Source: three-view drawing plus pictorial views. Frame: mm from the lowest corner of the part. A direction names the side the tool comes from. Give positions to 0.01 mm unless a question says otherwise; leave off trailing zeros. Order: outer loops, then holes, each group sorted by start corner. A loop starts at its lowest first (then second) coordinate and runs counter-clockwise, first axis right, second up.
1) Section D-D, the plane x = 21. Return loops of the section in (y, z), plus the area to 3 significant figures.
2) Access query for the marked faces 1 and 2. Directions: +Z, -Z, +X, -X, +Y, -Y. A direction counts if a zero-diameter tool reaches every point of the face in a straight line with its end or side. Return the directions, or none.
3) Section A-A, the plane x = 36. Return loops of the section in (y, z), plus the area to 3 significant figures.
4) Material intervals for line 1 (Z direction, x = 41, y = 54.5); line 2 (X direction, y = 53.5, z = 17.5); line 3 (X direction, y = 11.5, z = 25), sorted ascending.
5) Section C-C, the plane z = 11. Return loops of the section in (x, y), plus the area to 3 significant figures.
6) Section B-B, the plane y = 60. Return loops of the section in (x, z), plus the area to 3 significant figures.
7) First-contact query: P1, Ø2, axis at x = 9, y = 84, coming from the -Z side; P2, Ø1, axis at x = 26.5, z = 30, coming from the -Y side; P3, Ø1, axis at y = 79, z = 42.5, coming from the +X side; P4, Ø6, axis at y = 79, z = 32, coming from the +X side. Flat tips, straight axial feed; report the tip coordinate or a pass-through.
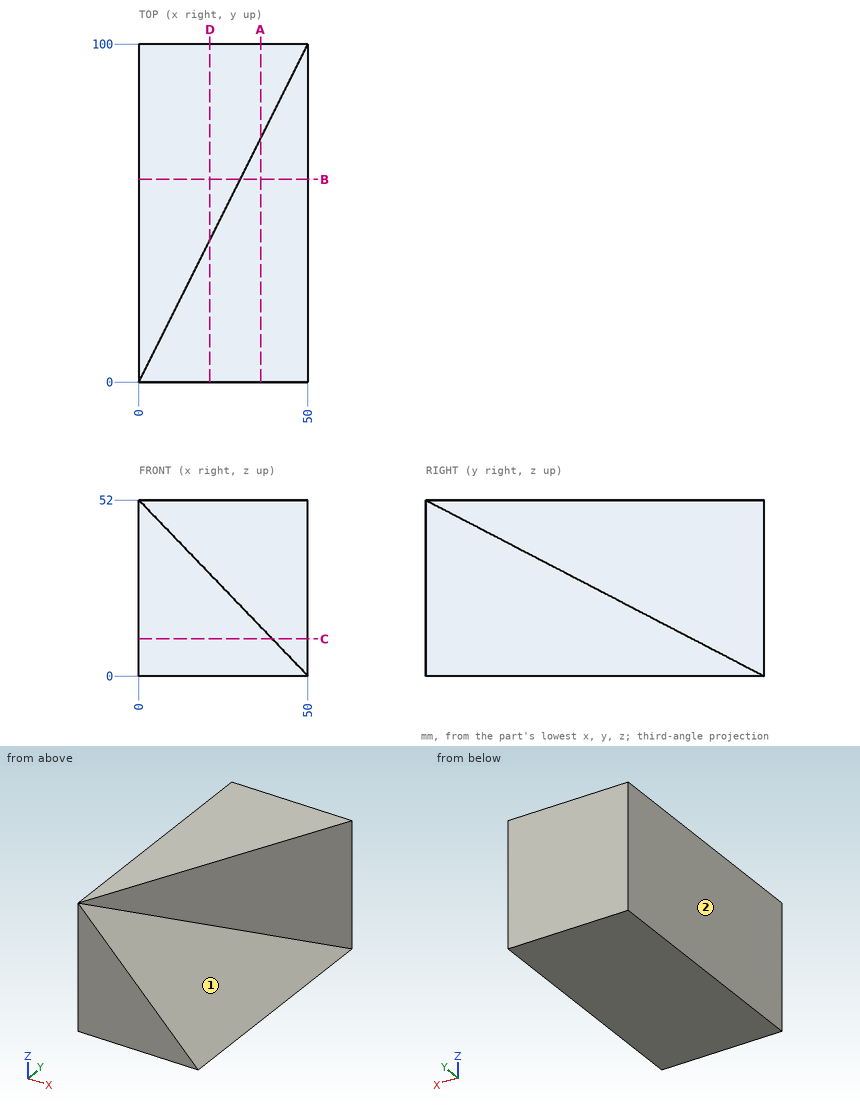
From the geometry:
1. outline: (0, 0) - (100, 0) - (100, 52) - (42, 52) - (42, 30.16) - (0, 30.16) - close
1. area: 4,280 mm2
2. face 1: +Z, +X, -Y
2. face 2: +Z, -Z, -X, +Y, -Y
3. outline: (0, 0) - (100, 0) - (100, 52) - (72, 52) - (72, 14.56) - (0, 14.56) - close
3. area: 2,500 mm2
4. line 1: z = 0 to 9.36
4. line 2: x = 0 to 33.17
4. line 3: x = 0 to 25.96
5. outline: (0, 0) - (39.42, 0) - (39.42, 78.85) - (50, 100) - (0, 100) - close
5. area: 4,050 mm2
6. outline: (0, 0) - (50, 0) - (30, 20.8) - (30, 52) - (0, 52) - close
6. area: 1,770 mm2
7. P1: stops at z = 0
7. P2: stops at y = 52
7. P3: stops at x = 39.75
7. P4: stops at x = 41
